Source: CAD feature listing. Evaluate the final solid. Frame: model axes, mm. A direction names the side the tool comes from. Round coordinates to 2 decimals unless told otherwise and drop trailing zeros. Loops run counter-clockwise (first coordinate to the right, second up) from the corner with the lowest first, then second, coordinate; pieces in that order, holes last. Notation, with made-up numbers: (36.25, -10) - (53.25, -10) arc R19 cw to (53.25, -2) - close; hole circle Ø4 at (81, 55.25). An arc over 180 degrees is marked (long way). Write item = value, one per line. Start each with the question number.
Autodesk Inventor part; units mm, degrees
ref_plane "YZ Plane" through (0, 0, 0) normal (1, 0, 0) x (0, 1, 0)
ref_plane "XZ Plane" through (0, 0, 0) normal (0, 1, 0) x (-1, 0, 0)
ref_plane "XY Plane" through (0, 0, 0) normal (0, 0, 1) x (1, 0, 0)
sketch "Sketch1" plane through (0, 0, 0) normal (0, 0, 1) x (1, 0, 0)
  circle A0 centre (0, 0) radius 5.625
  circle A1 centre (0, 0) radius 7.375
  dimension "d0" = 11.25
  dimension "d1" = 14.75
extrude "Extrusion1" add sketch "Sketch1" along normal blind 9
sketch "Sketch2" plane through (0, 0, 9) normal (0, 0, 1) x (1, 0, 0)
  circle A0 centre (0, 0) radius 7.375
  circle A1 centre (0, 0) radius 7.375
extrude "Extrusion2" add sketch "Sketch2" along normal blind 17.5
sketch "Sketch3" plane through (0, 0, 26.5) normal (0, 0, 1) x (1, 0, 0)
  circle A0 centre (0, 0) radius 7.375
  circle A1 centre (0, 0) radius 3.575
  dimension "d6" = 7.15
extrude "Extrusion3" cut sketch "Sketch3" against normal blind 7.5 contours A1
sketch "Sketch4" plane through (0, 0, 19) normal (0, 0, 1) x (1, 0, 0)
  circle A0 centre (0, 0) radius 3.575
  circle A1 centre (0, 0) radius 3.575
extrude "Extrusion4" cut sketch "Sketch4" against normal blind 3.2
chamfer "Chamfer1" distance 3.575 angle 45 1 edges at (-3.575, 0, 15.8)
sketch "Sketch5" plane through (0, 0, 9) normal (0, 0, -1) x (-1, 0, 0)
  circle A0 centre (0, 0) radius 5.625
  line L0 (-0.6, 5.5929) -> (0, 4.125)
  line L1 (0, 4.125) -> (0.6, 5.5929)
  arc A1 (0.6, 5.5929) -> (-0.6, 5.5929) centre (0, 0) ccw
  line L2 (-3.3161, 4.5436) -> (-2.0625, 3.5724)
  line L3 (-2.0625, 3.5724) -> (-2.2768, 5.1436)
  arc A2 (-2.2768, 5.1436) -> (-3.3161, 4.5436) centre (0, 0) ccw
  line L4 (-5.1436, 2.2768) -> (-3.5724, 2.0625)
  line L5 (-3.5724, 2.0625) -> (-4.5436, 3.3161)
  arc A3 (-4.5436, 3.3161) -> (-5.1436, 2.2768) centre (0, 0) ccw
  line L6 (-5.5929, -0.6) -> (-4.125, 0)
  line L7 (-4.125, 0) -> (-5.5929, 0.6)
  arc A4 (-5.5929, 0.6) -> (-5.5929, -0.6) centre (0, 0) ccw
  line L8 (-4.5436, -3.3161) -> (-3.5724, -2.0625)
  line L9 (-3.5724, -2.0625) -> (-5.1436, -2.2768)
  arc A5 (-5.1436, -2.2768) -> (-4.5436, -3.3161) centre (0, 0) ccw
  line L10 (-2.2768, -5.1436) -> (-2.0625, -3.5724)
  line L11 (-2.0625, -3.5724) -> (-3.3161, -4.5436)
  arc A6 (-3.3161, -4.5436) -> (-2.2768, -5.1436) centre (0, 0) ccw
  line L12 (0.6, -5.5929) -> (0, -4.125)
  line L13 (0, -4.125) -> (-0.6, -5.5929)
  arc A7 (-0.6, -5.5929) -> (0.6, -5.5929) centre (0, 0) ccw
  line L14 (3.3161, -4.5436) -> (2.0625, -3.5724)
  line L15 (2.0625, -3.5724) -> (2.2768, -5.1436)
  arc A8 (2.2768, -5.1436) -> (3.3161, -4.5436) centre (0, 0) ccw
  line L16 (5.1436, -2.2768) -> (3.5724, -2.0625)
  line L17 (3.5724, -2.0625) -> (4.5436, -3.3161)
  arc A9 (4.5436, -3.3161) -> (5.1436, -2.2768) centre (0, 0) ccw
  line L18 (5.5929, 0.6) -> (4.125, 0)
  line L19 (4.125, 0) -> (5.5929, -0.6)
  arc A10 (5.5929, -0.6) -> (5.5929, 0.6) centre (0, 0) ccw
  line L20 (4.5436, 3.3161) -> (3.5724, 2.0625)
  line L21 (3.5724, 2.0625) -> (5.1436, 2.2768)
  arc A11 (5.1436, 2.2768) -> (4.5436, 3.3161) centre (0, 0) ccw
  line L22 (2.2768, 5.1436) -> (2.0625, 3.5724)
  line L23 (2.0625, 3.5724) -> (3.3161, 4.5436)
  arc A12 (3.3161, 4.5436) -> (2.2768, 5.1436) centre (0, 0) ccw
  point P0 (0, 5.625)
  point P1 (-2.8125, 4.8714)
  point P2 (-4.8714, 2.8125)
  point P3 (-5.625, 0)
  point P4 (-4.8714, -2.8125)
  point P5 (-2.8125, -4.8714)
  point P6 (0, -5.625)
  point P7 (2.8125, -4.8714)
  point P8 (4.8714, -2.8125)
  point P9 (5.625, 0)
  point P10 (4.8714, 2.8125)
  point P11 (2.8125, 4.8714)
  dimension "d16" = 1.5
  dimension "d17" = 0.6
  dimension "d18" = 0
  dimension "d19" = 0
  dimension "d20" = 0.6
  dimension "d23" = 360
extrude "Extrusion5" add sketch "Sketch5" along normal blind 9 contours A0 L19 L18 | L21 L20 A0 | A0 L17 L16 | L23 L22 A0 | A0 L15 L14 | L1 L0 A0 | A0 L13 L12 | L3 L2 A0 | A0 L11 L10 | L5 L4 A0 | A0 L9 L8 | L7 L6 A0
properties part number "shaft coupler"
(1) Cut plane C-C (y = -6.25). Output: boundary loops of the cut face in (x, z).
(2) Pin query (flat end, axial travel): P1, Ø3, axis at x = 4, z = 4.5, coming from the -Y side; P2, Ø4, axis at x = -6, z = 13, coming from the +Y side; P3, Ø8, axis at y = -4.5, z = 14, coming from the -X side. Return the tip coordinate at first contact, or that it passes through.
(3) Material intervals for line 1 along Y through (x, z) = (0, 22) (3 decimals); line 2 along X through (y, z) = (0.25, 24.25); line 3 along Y through (x, z) = (-4, 1.5), sorted ascending. Write a range as from..to.
(4) Cut plane A-A (z = 24). Output: boundary loops of the cut face in (x, y) (3 decimals), and give its area (3 significant figures).
(5) Mould query, pull axis X, two halves, no side actions, for faces 3 (the face through (4.849, 0.296, 4.563)), 4 (the face through (0, -5, 0)). Classes: +X half, -X half, draft (parallel to the pull), parting line (faces both ways), or undercut.
(6) Cut plane B-B (x = 6). Output: boundary loops of the cut face in (y, z), and give its area (3 significant figures).
(7) Access query for faces 1 (the face through (-2.17, 4.37, 4.56)), 2 (the face through (0.47, -0.903, 16.818)). Directions: +Z, -Z, +X, -X, +Y, -Y. A direction counts if a zero-diameter tool reaches every point of the face in a straight line with its end or side. Return the directions, or none.
Solution:
q1.outline = (-3.92, 0) - (3.92, 0) - (3.92, 26.5) - (-3.92, 26.5) - close
q2.P1 = -6.94
q2.P2 = 6.2
q2.P3 = -7.36
q3.line_1 = -7.375..-3.575, 3.575..7.375
q3.line_2 = -7.37..-3.57, 3.57..7.37
q3.line_3 = -6.2..-3.95, -2.61..-2.12, 2.12..2.61, 3.95..6.2
q4.outline = circle Ø14.75 at (0, 0); hole circle Ø7.15 at (0, 0)
q4.area = 131 mm^2
q5.face_3 = undercut
q5.face_4 = draft
q6.outline = (-4.29, 0) - (4.29, 0) - (4.29, 26.5) - (-4.29, 26.5) - close
q6.area = 227 mm^2
q7.face_1 = -Z
q7.face_2 = +Z
